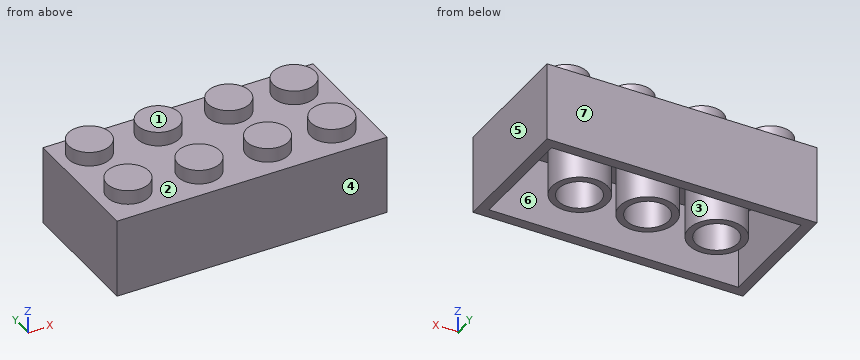
```python
from build123d import *

# Parameters (mm, degrees)
F0_W     = 31.3436
F0_H     = 9.144
F1_DEPTH = 15.367
F2_R     = 2.4384
F3_DEPTH = 1.651
F4_T     = -1.1938
F5_R     = 3.2258
F6_DEPTH = 7.88406
F7_R     = 2.4384
F8_DEPTH = 8.37132


# Not quite as in the source:
# - the program builds the solid bodies; features that only make, move or delete a surface that nothing else refers to are left out


with BuildPart() as f1:
    # F0 (on Front) → F1 (new body)
    with BuildSketch(Plane.XZ):
        Rectangle(F0_W, F0_H)
    extrude(amount=F1_DEPTH)

    # F2 (on face) → F3 (join)
    with BuildSketch(Plane.XY.offset(4.572)):
        with Locations((-12.0193809271, -3.087217221)):
            Circle(F2_R)
        with Locations((-4.1364012286, -3.2935778145)):
            Circle(F2_R)
        with Locations((4.0354835801, -3.33484984)):
            Circle(F2_R)
        with Locations((11.5470141172, -3.4586666152)):
            Circle(F2_R)
        with Locations((11.4644700661, -11.4241903648)):
            Circle(F2_R)
        with Locations((4.0767556056, -11.3003747538)):
            Circle(F2_R)
        with Locations((-3.9300406352, -11.3829188049)):
            Circle(F2_R)
        with Locations((-12.0193809271, -11.094013229)):
            Circle(F2_R)
    extrude(amount=F3_DEPTH)

    # F4
    f4_openings = [f1.faces().sort_by_distance(p)[0] for p in [
        (0, -7.6835, -4.572),
    ]]
    offset(amount=F4_T, openings=f4_openings, kind=Kind.INTERSECTION)

    # F5 (on face) → F6 (join)
    with BuildSketch(Plane(origin=(0, 0, 3.3782), x_dir=(1, 0, 0), z_dir=(0, 0, -1))):
        with Locations((-8.1251291558, 7.3120272718)):
            Circle(F5_R)
        with Locations((0, 7.1467519738)):
            Circle(F5_R)
        with Locations((7.7412822284, 7.3671187274)):
            Circle(F5_R)
    extrude(amount=F6_DEPTH)

    # F7 (on face) → F8 (cut)
    with BuildSketch(Plane(origin=(0, 0, -4.50586), x_dir=(1, 0, 0), z_dir=(0, 0, -1))):
        with Locations((-8.1251291558, 7.3120272718)):
            Circle(F7_R)
        with Locations((-0.012788114, 7.1699875407)):
            Circle(F7_R)
        with Locations((7.7589382418, 7.4168494903)):
            Circle(F7_R)
    extrude(amount=-F8_DEPTH, mode=Mode.SUBTRACT)


solid = f1.part
```
Read the model definition and answer for the solid it produces. Units are mm, in the model's axes. Face numbers are marked on the shaded views. A direction names the side the tool comes from. Round coordinates to 2 decimals unless told otherwise and drop trailing zeros. Write each loop counter-clockwise with the first axis right and the second up, starting at its lowest first coordinate (ties: lowest second). Pieces come first, ordered by that corner, then holes. Notation, with made-up numbers: (-24, 71.5) -> (8, 71.5) arc R15 cw to (8, 86.5) -> close; hole circle Ø7 at (51, 32). An arc over 180 degrees is marked (long way). Answer in a Markdown table with one row per item. Add a question column.
1) Determine the mould class of the marked faces 4, 5, 6 and 7 for opening direction Y: pulls with the +Y half, pulls with the -Y half, needs draft (parallel to the pull), parting line crosses it, or undercut.
2) Find section A-A, the plane z = 1. Determine the outline of the cut face in (x, y), and give its area (3 significant figures).
3) Find section C-C, the plane z = 5.5. Determine the outline of the cut face in (x, y).
4) Find section B-B, the plane x = -8. Determine the outline of the cut face in (y, z), and give its area (3 significant figures).
5) Given P1, Ø5, axis at x = -8.5, y = -7.5, coming from the -Z side; P2, Ø0.7, axis at x = -4.5, y = -3.5, coming from the -Z side; P3, Ø1.9, axis at x = 7.5, y = -6.5, coming from the -Z side, each flat-ended and moving along its own axis, determine where each tip first touches the part or whether it passes through.
6) Which of the six approach directions +Z, -Z, +X, -X, +Y, -Y give full straight-line access (tool end or side, diameter ignored) to the marked faces 1, 2 and 3?
7) Find section D-D, the plane x = 0. Determine the outline of the cut face in (y, z).
8) Consider line 1 (Y direction, x = -4, z = 3.5); line 2 (X direction, y = -2.5, z = 2); line 3 (Y direction, x = 12, z = 1.25). Determine where each line is inside the solid, lowest interval first.
Findings below:
| question | item | result |
|---|---|---|
| 1 | face 4 | pulls with the -Y half |
| 1 | face 5 | needs draft |
| 1 | face 6 | undercut |
| 1 | face 7 | pulls with the +Y half |
| 2 | outline | (-15.67, -15.37) -> (15.67, -15.37) -> (15.67, 0) -> (-15.67, 0) -> close; circle Ø6.45 at (-8.13, -7.31); circle Ø6.45 at (0, -7.15); circle Ø6.45 at (7.74, -7.37); hole (-14.48, -14.17) -> (14.48, -14.17) -> (14.48, -1.19) -> (-14.48, -1.19) -> close; hole circle Ø4.88 at (-8.13, -7.31); hole circle Ø4.88 at (-0.01, -7.17); hole circle Ø4.88 at (7.76, -7.42) |
| 2 | area | 148 mm² |
| 3 | outline | circle Ø4.88 at (-12.02, -11.09); circle Ø4.88 at (-12.02, -3.09); circle Ø4.88 at (-4.14, -3.29); circle Ø4.88 at (-3.93, -11.38); circle Ø4.88 at (4.04, -3.33); circle Ø4.88 at (4.08, -11.3); circle Ø4.88 at (11.46, -11.42); circle Ø4.88 at (11.55, -3.46) |
| 4 | outline | (-15.37, -4.57) -> (-14.17, -4.57) -> (-14.17, 3.38) -> (-10.54, 3.38) -> (-10.54, -4.51) -> (-9.75, -4.51) -> (-9.75, 3.87) -> (-4.88, 3.87) -> (-4.88, -4.51) -> (-4.09, -4.51) -> (-4.09, 3.38) -> (-1.19, 3.38) -> (-1.19, -4.57) -> (0, -4.57) -> (0, 4.57) -> (-15.37, 4.57) -> close |
| 4 | area | 47.4 mm² |
| 5 | P1 | z = -4.51 |
| 5 | P2 | z = 5.03 |
| 5 | P3 | z = 3.87 |
| 6 | face 1 | +Z, +X, -X, +Y, -Y |
| 6 | face 2 | +Z |
| 6 | face 3 | -Z |
| 7 | outline | (-15.37, -4.57) -> (-14.17, -4.57) -> (-14.17, 3.38) -> (-10.37, 3.38) -> (-10.37, -4.51) -> (-9.61, -4.51) -> (-9.61, 3.87) -> (-4.73, 3.87) -> (-4.73, -4.51) -> (-3.92, -4.51) -> (-3.92, 3.38) -> (-1.19, 3.38) -> (-1.19, -4.57) -> (0, -4.57) -> (0, 4.57) -> (-15.37, 4.57) -> close |
| 8 | line 1 | -15.37 to -12.63, -10.14 to -4.53, -2.06 to 0 |
| 8 | line 2 | -15.67 to -14.48, 14.48 to 15.67 |
| 8 | line 3 | -15.37 to -14.17, -1.19 to 0 |
